Part model, mm, in its own coordinate system. A direction names the side the tool comes from. Coordinates: 2 decimals unless noted, no trailing zeros. Write each loop counter-clockwise with the first axis right and the second up, starting at its lowest first coordinate (ties: lowest second). Pieces come first, ordered by that corner, then holes. Notation, with made-up numbers: (87.5, 10.25) -> (119.5, 10.25) arc R23 cw to (119.5, 26.25) -> close; hole circle Ø9 at (18.25, -9). An arc over 180 degrees is marked (long way). Write item = value, one per line. Start each with the question number.
Q1. Pin check, flat tips, straight feed: P1, Ø12, axis at y = -6.5, z = 10.5, coming from the -X side; P2, Ø12, axis at y = -11.5, z = 4, coming from the +X side (3 decimals); P3, Ø2, axis at x = 17, z = 4, coming from the -Y side; P4, Ø8, axis at y = -18, z = 10, coming from the -X side. Stop position of each tip, or through.
Q2. Tool access for faces 1 (the flat face through (7.4, 0, -3.6)), 2 (the cylindrical face through (-1.93, -47.37, -8.68)): list every direction of +Z, -Z, +X, -X, +Y, -Y with a clear straight run to the whole face (end or side of a thin tool).
Q3. Pull direction X, two halves, no side cores. Call faces 3 (the flat face through (7, -44.45, -7)), 4 (the cylindrical face through (-1.72, -26.3, -7.75)), 5 (the cylindrical face through (21.199, -21.985, 6.676)): released by +X, released by -X, zero draft, split by the parting line, or undercut.
Q4. Band-saw the part on A-A, the plane y = -48. List the corners of the cut face in (x, z) (1 decimal).
Q5. Probe line 1 (Z direction, x = 0, y = -17) (1 decimal); line 2 (Y direction, x = -12, z = 6); line 3 (Z direction, x = -5, y = -2.5). List the from-to ranges inside material, lowest first.
from build123d import *

# Parameters (mm, degrees)
F0_R     = 8.89
F0_R_2   = 7.9375
F1_DEPTH = 53.34
F0_R_3   = 22.225
F2_DEPTH = 44.45
F3_R     = 5.08
F4_R     = 5.08


# Not quite as in the source:
# - a fillet or chamfer that OpenCascade refuses, or shapes differently, is made with other operations: its cross-section is extruded or revolved along the edge and cut away or added


with BuildPart() as f1:
    # F0 (on Front) → F1 (new body)
    with BuildSketch(Plane.XZ):
        Circle(F0_R)
        Circle(F0_R_2, mode=Mode.SUBTRACT)
    extrude(amount=F1_DEPTH)

    # F0 (on Front) → F2 (join)
    with BuildSketch(Plane.XZ):
        Circle(F0_R_3)
        Circle(F0_R, mode=Mode.SUBTRACT)
    extrude(amount=F2_DEPTH)

    # F3
    f3_edges = [f1.edges().sort_by_distance(p)[0] for p in [
        (-22.225, -44.45, 0),
    ]]
    fillet(f3_edges, radius=F3_R)

    # F4
    f4_edges = [f1.edges().sort_by_distance(p)[0] for p in [
        (-22.225, 0, 0),
    ]]
    fillet(f4_edges, radius=F4_R)

    # F5: fillet of radius 5.08 on 1 edges, made by hand

    # F5_s1 → F5_t2 (revolve, cut)
    with BuildSketch(Plane.XY):
        with BuildLine():
            ThreePointArc((8.89, -50.3785571506), (8.6460159222, -51.9339831373), (7.9375, -53.34))
            Line((7.9375, -53.34), (8.89, -53.34))
            Line((8.89, -53.34), (8.89, -50.3785571506))
        make_face()
    revolve(axis=Axis((0, -53.34, 0), (0, -1, 0)), mode=Mode.SUBTRACT)


solid = f1.part
Ans:
q1.P1 = -21.76
q1.P2 = 22.225
q1.P3 = -44.45
q1.P4 = -21.4
q2.face_1 = +Z, -Z, +X, -X, +Y
q2.face_2 = -Y
q3.face_3 = zero draft
q3.face_4 = undercut
q3.face_5 = split by the parting line
q4.outline = circle Ø17.8 at (0, 0); hole circle Ø15.9 at (0, 0)
q5.line_1 = -22.2 to -7.9, 7.9 to 22.2
q5.line_2 = -44.45 to 0
q5.line_3 = -20.93 to -6.16, 6.16 to 20.93
